from build123d import *

# Parameters (mm, degrees)
F0_R     = 53.5
F0_R_2   = 50.5
F1_DEPTH = 6
F3_DEPTH = 3


with BuildPart() as f1:
    # F0 (on Top) → F1 (new body)
    with BuildSketch(Plane.XY):
        Circle(F0_R)
        Circle(F0_R_2, mode=Mode.SUBTRACT)
    extrude(amount=F1_DEPTH)

    # F2 (on Top) → F3 (join)
    with BuildSketch(Plane.XY):
        with BuildLine():
            ThreePointArc((14.851876, -51.397196), (0, -53.5), (-14.851876, -51.397196))
            ThreePointArc((-14.851876, -51.397196), (0, -68.5), (14.851876, -51.397196))
        make_face()
        with BuildLine():
            ThreePointArc((-14.851876, 51.397196), (0, 53.5), (14.851876, 51.397196))
            ThreePointArc((14.851876, 51.397196), (0, 68.5), (-14.851876, 51.397196))
        make_face()
    extrude(amount=F3_DEPTH)


solid = f1.part
Design review of the part built by this model. Coordinates are the model's own, in mm. Coordinates: 2 decimals unless noted, no trailing zeros. Order: outer loops, then holes, each group sorted by start corner. A loop starts at its lowest first (then second) coordinate and runs counter-clockwise, first axis right, second up.
Item 1: For pin 1 Ø5 at (x, y) = (2, -62.5) entering from +Z; pin 2 Ø12 at (x, y) = (34, 30) entering from -Z; pin 3 Ø1 at (x, z) = (28, 3.5) entering from +Y, all flat-tipped, find the tip position at first contact; note any pin that passes through.
Item 2: For line 1 (Y direction, x = 0, z = 1.8); line 2 (X direction, y = 1, z = 5.5); line 3 (Y direction, x = 25.5, z = 2), list the stretches that pass through material, from the lowest coordinate up.
Item 3: Take a section at C-C, the plane z = 4.25. Write out the cut boundary in (x, y).
Item 4: Take a section at A-A, the plane y = 0. Write out the cut boundary in (x, z).
Item 5: Take a section at B-B, the plane x = -43. Write out the cut boundary in (y, z), then the cut area to 3 significant figures.
Item 6: Take a section at D-D, the plane x = -2. Write out the cut boundary in (y, z), then the cut area to 3 significant figures.
Item 7: The part is to be moulded in two halves that separate along X. For faces 1 (the cylindrical face through (-0.359, -68.496, 1.479)), 2 (the flat face through (7.7, -50.4, 0)), 3 (the cylindrical face through (-10.95, -49.3, 2.96)), say which applies: pulls with the +X half, pulls with the -X half, needs draft (parallel to the pull), parting line crosses it, or undercut.
The answers:
1. pin 1: stops at z = 3
1. pin 2: stops at z = 0
1. pin 3: stops at y = 45.89
2. line 1: y = -68.5 to -50.5, 50.5 to 68.5
2. line 2: x = -53.49 to -50.49, 50.49 to 53.49
2. line 3: y = -47.03 to -43.59, 43.59 to 47.03
3. outline: circle Ø107 at (0, 0); hole circle Ø101 at (0, 0)
4. outline: (-53.5, 0) - (-50.5, 0) - (-50.5, 6) - (-53.5, 6) - close; (50.5, 0) - (53.5, 0) - (53.5, 6) - (50.5, 6) - close
5. outline: (-31.83, 0) - (-26.48, 0) - (-26.48, 6) - (-31.83, 6) - close; (26.48, 0) - (31.83, 0) - (31.83, 6) - (26.48, 6) - close
5. area: 64.2 mm2
6. outline: (-68.37, 0) - (-50.46, 0) - (-50.46, 6) - (-53.46, 6) - (-53.46, 3) - (-68.37, 3) - close; (50.46, 0) - (68.37, 0) - (68.37, 3) - (53.46, 3) - (53.46, 6) - (50.46, 6) - close
6. area: 125 mm2
7. face 1: parting line crosses it
7. face 2: needs draft
7. face 3: undercut
